```python
from build123d import *

# Parameters (mm, degrees)
BASENUTSKE_R  = 3.96875
BASENUT_DEPTH = 8.5598


with BuildPart() as part:
    # BaseNutSke → BaseNut (new body)
    with BuildSketch(Plane.XY):
        Polygon((7.1374, 4.120779811), (7.1374, -4.120779811), (0, -8.241559623), (-7.1374, -4.120779811), (-7.1374, 4.120779811), (0, 8.241559623), align=None)
        Circle(BASENUTSKE_R, mode=Mode.SUBTRACT)
    extrude(amount=-BASENUT_DEPTH)

    # Sketch3 → Double-Chamfer (revolve, cut)
    with BuildSketch(Plane(origin=(0, 0, 0), x_dir=(0, 0, -1), z_dir=(1, 0, 0))):
        Polygon((8.5598, 7.1374), (7.527798, 8.241559623), (7.527798, 20.941559623), (21.2598, 20.941559623), (21.2598, 7.1374), align=None)
        Polygon((1.032002, 20.941559623), (-12.7, 20.941559623), (-12.7, 7.1374), (0, 7.1374), (1.032002, 8.241559623), align=None)
    revolve(axis=Axis((0, 0, 0), (0, 0, -1)), mode=Mode.SUBTRACT)

    # Sketch5 → EndChamfer (revolve, cut)
    with BuildSketch(Plane(origin=(0, 0, 0), x_dir=(0, 0, -1), z_dir=(1, 0, 0))):
        Polygon((8.5344, 5.16001), (7.616857845, 3.849624), (8.5852, 3.849624), (8.5852, 5.16001), align=None)
        Polygon((-0.0508, 5.16001), (0, 5.16001), (0.917542155, 3.849624), (-0.0508, 3.849624), align=None)
    revolve(axis=Axis((0, 0, -25.037505729), (0, 0, -1)), mode=Mode.SUBTRACT)


solid = part.part
```
CAD build for the part. Positions are in the model's coordinates, mm. Give positions to 0.01 mm unless a question says otherwise; leave off trailing zeros. Order: outer loops, then holes, each group sorted by start corner. A loop starts at its lowest first (then second) coordinate and runs counter-clockwise, first axis right, second up.
(1) Saw through at B-B, the plane z = -8. Give the cut face in (x, y).
(2) Flat gauge pins, fed straight in: pin 1 (7 mm diameter, centred on x = 0, y = 0, fed in from -Z); pin 2 (2 mm diameter, centred on x = 1.5, z = -3.5, fed in from -Y); pin 3 (3 mm diameter, centred on x = 3.5, z = -7, fed in from -Y); pin 4 (5 mm diameter, centred on x = -5, z = -3, fed in from +Y). Where does each tip first touch, or does it go through?
(3) Drill centre lines: L1, parallel to Y at x = 2.75, z = -1.75; L2, parallel to Y at x = 0, z = -8.5; L3, parallel to X at y = 2.25, z = -3.75. Where is each one in solid material? Low to high.
(4) Saw through at A-A, the plane z = -5. Give the cut face in (x, y), then the cut area to 3 significant figures.
(5) Mould opens along X. For faces 1 (the conical face through (6.42, -3.69, -0.25)), 2 (the flat face through (-7.137, 0, -4)), 3 (the cylindrical face through (3.785, 1.192, -4.219)), 4 (the conical face through (-0.018, 7.406, -8.309)) say: released by +X, released by -X, zero draft, split by the parting line, or undercut.
Results found:
1. outline: (-7.14, -2.98) arc R7.74 ccw to (-6.15, -4.69) - (-0.98, -7.67) arc R7.74 ccw to (0.98, -7.67) - (6.15, -4.69) arc R7.74 ccw to (7.14, -2.98) - (7.14, 2.98) arc R7.74 ccw to (6.15, 4.69) - (0.98, 7.67) arc R7.74 ccw to (-0.98, 7.67) - (-6.15, 4.69) arc R7.74 ccw to (-7.14, 2.98) - close; hole circle Ø8.79 at (0, 0)
2. pin 1: passes through
2. pin 2: stops at y = -7.95
2. pin 3: stops at y = -7.09
2. pin 4: stops at y = 6.8
3. L1: y = -6.65 to -2.86, 2.86 to 6.65
3. L2: y = -7.2 to -5.11, 5.11 to 7.2
3. L3: x = -7.14 to -3.27, 3.27 to 7.14
4. outline: (-7.14, -4.12) - (0, -8.24) - (7.14, -4.12) - (7.14, 4.12) - (0, 8.24) - (-7.14, 4.12) - close; hole circle Ø7.94 at (0, 0)
4. area: 127 mm2
5. face 1: released by +X
5. face 2: released by -X
5. face 3: undercut
5. face 4: split by the parting line
